The model under review builds one solid part; all positions refer to its coordinate system, in mm. Face numbers are marked on the shaded views. A direction names the side the tool comes from. Coordinates: 2 decimals unless noted, no trailing zeros. Order: outer loops, then holes, each group sorted by start corner. A loop starts at its lowest first (then second) coordinate and runs counter-clockwise, first axis right, second up.
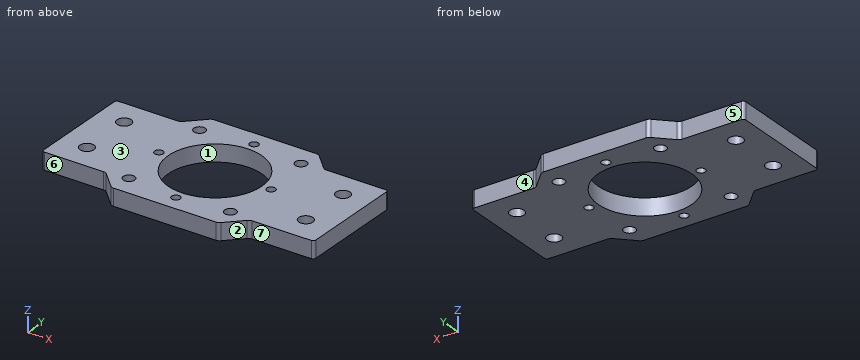
Autodesk Inventor part; units mm, degrees
ref_plane "YZ Plane" through (0, 0, 0) normal (1, 0, 0) x (0, 1, 0)
ref_plane "XZ Plane" through (0, 0, 0) normal (0, 1, 0) x (-1, 0, 0)
ref_plane "XY Plane" through (0, 0, 0) normal (0, 0, 1) x (1, 0, 0)
sketch "Sketch1" plane through (0, 0, 0) normal (0, 0, 1) x (1, 0, 0)
  line L0 (51, -20) -> (-51, -20)
  line L1 (-51, -20) -> (-51, 20)
  line L2 (-51, 20) -> (51, 20)
  line L3 (51, 20) -> (51, -20)
  line L4 (51, -20) -> (-51, 20) construction
  line L5 (-51, -20) -> (51, 20) construction
  line L6 (21, -21) -> (-21, -21) construction
  line L7 (-21, -21) -> (-21, 21) construction
  line L8 (-21, 21) -> (21, 21) construction
  line L9 (21, 21) -> (21, -21) construction
  line L10 (21, -21) -> (-21, 21) construction
  line L11 (-21, -21) -> (21, 21) construction
  line L12 (29.6985, 0) -> (0, 29.6985) construction
  line L13 (0, 29.6985) -> (-29.6985, 0) construction
  line L14 (-29.6985, 0) -> (0, -29.6985) construction
  line L15 (0, -29.6985) -> (29.6985, 0) construction
  line L16 (29.6985, 0) -> (-29.6985, 0) construction
  line L17 (0, 29.6985) -> (0, -29.6985) construction
  circle A0 centre (0, 0) radius 26 construction
  line L18 (20, -27) -> (-20, -27)
  line L19 (-27, -20) -> (-27, 20)
  line L20 (-20, 27) -> (20, 27)
  line L21 (27, 20) -> (27, -20)
  line L22 (27, -27) -> (-27, 27) construction
  line L23 (-27, -27) -> (27, 27) construction
  line L24 (24.4641, -27) -> (17.5359, -27)
  line L25 (-27, 20) -> (-20, 27)
  line L26 (20, 27) -> (27, 20)
  line L27 (20, -27) -> (27, -20)
  line L28 (-20, -27) -> (-27, -20)
  circle A1 centre (-21, 21) radius 3.5355
  point P0 (28.5056, -20)
  point P1 (27, 20)
  point P2 (27, -20)
  point P3 (27, 20)
  point P4 (-27, -20)
  point P5 (27, -20)
  point P6 (-27, -20)
  dimension "d0" = 102
  dimension "d1" = 40
  dimension "d2" = 42
  dimension "d3" = 42
  dimension "d4" = 42
  dimension "d5" = 42
  dimension "d6" = 52
  dimension "d8" = 54
  dimension "d43" = 7
  dimension "d44" = 7
  dimension "d45" = 7
  dimension "d46" = 7
  dimension "d47" = 7
  dimension "d48" = 7
  dimension "d49" = 7
  dimension "d50" = 7
  dimension "d51" = 7
  dimension "d52" = 6
  dimension "d53" = 6
extrude "Extrusion1" add sketch "Sketch1" along normal blind 6.35
fillet "Fillet1" radius 1 4 edges at (-51, 20, 3.175) (-51, -20, 3.175) (51, 20, 3.175) (51, -20, 3.175)
fillet "Fillet2" radius 2 8 edges at (-20, -27, 3.175) (-20, 27, 3.175) (20, 27, 3.175) (20, -27, 3.175) (-27, -20, 3.175) (-27, 20, 3.175) (27, -20, 3.175) (27, 20, 3.175)
sketch "Sketch2" plane through (0, 0, 6.35) normal (0, 0, 1) x (1, 0, 0)
  circle A0 centre (0, 0) radius 17.5
  dimension "d13" = 35
extrude "Extrusion2" cut sketch "Sketch2" against normal through all
sketch "Sketch3" plane through (0, 0, 6.35) normal (0, 0, 1) x (1, 0, 0)
  circle A0 centre (0, 0) radius 21 construction
  circle A1 centre (0, 0) radius 17.5
  line L0 (0, -21) -> (21, 0) construction
  line L1 (21, 0) -> (0, 21) construction
  line L2 (0, 21) -> (-21, 0) construction
  line L3 (-21, 0) -> (0, -21) construction
  line L4 (0, -21) -> (0, 21) construction
  line L5 (21, 0) -> (-21, 0) construction
  dimension "d17" = 42
hole "Hole1" at (0, 21, 6.35) at (21, 0, 6.35) at (0, -21, 6.35) at (-21, 0, 6.35) direction (0, 0, -1) diameter 3.242 end through all
sketch "Sketch4" plane through (0, 0, 6.35) normal (0, 0, 1) x (1, 0, 0)
  line L0 (41, -10) -> (-41, -10)
  line L1 (-41, -10) -> (-41, 10)
  line L2 (-41, 10) -> (41, 10)
  line L3 (41, 10) -> (41, -10)
  line L4 (41, -10) -> (-41, 10) construction
  line L5 (-41, -10) -> (41, 10) construction
  line L6 (-51, 19) -> (-51, -19)
  point P0 (0, 0)
  dimension "d25" = 20
  dimension "d26" = 10
hole "Hole2" at (-41, 10, 6.35) at (-41, -10, 6.35) at (41, 10, 6.35) at (41, -10, 6.35) direction (0, 0, -1) diameter 5.3 end through all
sketch "Sketch5" plane through (0, 0, 6.35) normal (0, 0, 1) x (1, 0, 0)
  line L0 (19, -19) -> (-19, -19)
  line L1 (-19, -19) -> (-19, 19)
  line L2 (-19, 19) -> (19, 19)
  line L3 (19, 19) -> (19, -19)
  line L4 (19, -19) -> (-19, 19) construction
  line L5 (-19, -19) -> (19, 19) construction
  point P0 (0, 0)
  dimension "d34" = 38
  dimension "d35" = 38
hole "Hole3" at (-19, 19, 6.35) at (19, 19, 6.35) at (19, -19, 6.35) at (-19, -19, 6.35) direction (0, 0, -1) diameter 4.3 end through all
equation "\"d44\" = d43"
equation "\"d45\" = d44"
equation "\"d46\" = d44"
equation "\"d47\" = d46"
equation "\"d48\" = d44"
equation "\"d49\" = d48"
equation "\"d50\" = d44"
equation "\"d51\" = d50"
equation "\"d53\" = d52"
properties part number "Z-Axis Motor Plate" material "Aluminum 6061"
(1) We need section C-C, the plane z = 4.75. Count the separate pieces of the cut face and the enclosed holes in it, and give its area (3 significant figures).
A:
separate pieces: 1
enclosed holes: 13
area: 3,600 mm2
(2) We need section B-B, the plane y = 4. Write out the cut boundary in (x, z).
A:
outline: (-51, 0) - (-17.04, 0) - (-17.04, 6.35) - (-51, 6.35) - close; (17.04, 0) - (51, 0) - (51, 6.35) - (17.04, 6.35) - close
(3) Draft analysis for pull direction X (two halves, no side actions). For the marked faces 1, 2 and 3, state which applies: released by +X, released by -X, zero draft, split by the parting line, or undercut.
A:
face 1: undercut
face 2: released by +X
face 3: zero draft
(4) Wall thickness on probe 1 along Y at (x, z) = (-41, 1); probe 2 along Y at (x, z) = (0, 5.25); probe 3 along Y at (x, z) = (-19, 2.25): over which ranges is each line inside the solid? List them lowest first.
A:
probe 1: y = -20 to -12.65, -7.35 to 7.35, 12.65 to 20
probe 2: y = -27 to -22.62, -19.38 to -17.5, 17.5 to 19.38, 22.62 to 27
probe 3: y = -27 to -21.15, -16.85 to 16.85, 21.15 to 27
(5) We need section D-D, the plane x = -42.5. Write out the cut boundary in (y, z).
A:
outline: (-20, 0) - (-12.18, 0) - (-12.18, 6.35) - (-20, 6.35) - close; (-7.82, 0) - (7.82, 0) - (7.82, 6.35) - (-7.82, 6.35) - close; (12.18, 0) - (20, 0) - (20, 6.35) - (12.18, 6.35) - close
(6) For pin 1 Ø3 at (x, y) = (0, -21) entering from +Z; pin 2 Ø1.5 at (x, z) = (23.5, 3) entering from +Y; pin 3 Ø1.9 at (x, z) = (-36.5, 3) entering from -Y, all flat-tipped, find the tip position at first contact; note any pin that passes through.
A:
pin 1: passes through
pin 2: stops at y = 24.25
pin 3: stops at y = -20
(7) Machinability: for the marked faces 4, 5, 6 and 7, which of the approach directions +Z, -Z, +X, -X, +Y, -Y give a long, thin tool a straight path to every point of the face, cutting with its end or side? Answer none if there is none.
A:
face 4: +Z, -Z, +X, +Y
face 5: +Z, -Z, -X, +Y
face 6: +Z, -Z, -X, -Y
face 7: +Z, -Z, +X, -Y
(8) We need section A-A, the plane x = 0. Write out the cut boundary in (y, z), and give its area (3 significant figures).
A:
outline: (-27, 0) - (-22.62, 0) - (-22.62, 6.35) - (-27, 6.35) - close; (-19.38, 0) - (-17.5, 0) - (-17.5, 6.35) - (-19.38, 6.35) - close; (17.5, 0) - (19.38, 0) - (19.38, 6.35) - (17.5, 6.35) - close; (22.62, 0) - (27, 0) - (27, 6.35) - (22.62, 6.35) - close
area: 79.5 mm2
